```python
from build123d import *

# Parameters (mm, degrees)
BOSS_EXTRUDE1_DEPTH = 2
CHAMFER1_SIZE       = 0.3


with BuildPart() as part:
    # Sketch1 → Boss-Extrude1 (new body)
    with BuildSketch(Plane(origin=(0, 0, 0), x_dir=(0, 0, -1), z_dir=(1, 0, 0))):
        with BuildLine():
            Line((3.968626967, 0.5), (6.982120022, 0.5))
            ThreePointArc((6.982120022, 0.5), (-7, 0), (6.982120022, -0.5))
            Line((6.982120022, -0.5), (3.968626967, -0.5))
            ThreePointArc((3.968626967, -0.5), (-4, 0), (3.968626967, 0.5))
        make_face()
    extrude(amount=BOSS_EXTRUDE1_DEPTH)

    # Chamfer1
    chamfer1_edges = [part.edges().sort_by_distance(p)[0] for p in [
        (2, 0, 4),
        (2, 0, 7),
        (0, 0, 4),
        (0, 0, 7),
    ]]
    chamfer(chamfer1_edges, length=CHAMFER1_SIZE)


solid = part.part
```
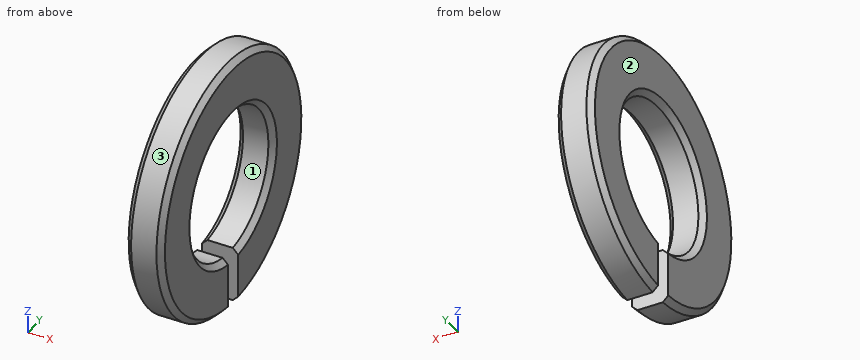
Source: CAD feature listing. Evaluate the final solid. Frame: model axes, mm. Face numbers are marked on the shaded views. Give positions to 0.01 mm unless a question says otherwise; leave off trailing zeros. Order: outer loops, then holes, each group sorted by start corner. A loop starts at its lowest first (then second) coordinate and runs counter-clockwise, first axis right, second up. Notation, with made-up numbers: (51.25, -12) -> (82.25, -12) arc R27 ccw to (82.25, 19) -> close; hole circle Ø4 at (7.25, 37.5). An arc over 180 degrees is marked (long way). Use a Markdown table: item, result.
Q1. Section A-A (z = 0). Return the cut outline in (x, y), and give its area (3 significant figures).
A:
| item | result |
|---|---|
| outline | (0, -6.7) -> (0.3, -7) -> (1.7, -7) -> (2, -6.7) -> (2, -4.3) -> (1.7, -4) -> (0.3, -4) -> (0, -4.3) -> close; (0, 4.3) -> (0.3, 4) -> (1.7, 4) -> (2, 4.3) -> (2, 6.7) -> (1.7, 7) -> (0.3, 7) -> (0, 6.7) -> close |
| area | 11.6 mm^2 |
Q2. Pull-direction query (Y, two-part tool) for the marked faces 1, 2 and 3; classes: +Y half, -Y half, draft (parallel to the pull), parting line (faces both ways), or undercut.
A:
| item | result |
|---|---|
| face 1 | undercut |
| face 2 | draft |
| face 3 | parting line |
Q3. Material intervals for line 1 (Y direction, x = 1, z = 0); line 2 (Y direction, x = 1.65, z = -1.25); line 3 (Z direction, x = 0.75, y = -6), sorted ascending. Write a range as [from, to].
A:
| item | result |
|---|---|
| line 1 | [-7, -4], [4, 7] |
| line 2 | [-6.89, -3.8], [3.8, 6.89] |
| line 3 | [-3.61, 3.61] |
Q4. Section B-B (y = 0). Return the cut outline in (x, z).
A:
| item | result |
|---|---|
| outline | (0, 4.3) -> (0.3, 4) -> (1.7, 4) -> (2, 4.3) -> (2, 6.7) -> (1.7, 7) -> (0.3, 7) -> (0, 6.7) -> close |
Q5. Section C-C (x = 1.2). Return the cut outline in (y, z).
A:
| item | result |
|---|---|
| outline | (-0.5, -6.98) -> (-0.5, -3.97) arc R4 cw (long way) to (0.5, -3.97) -> (0.5, -6.98) arc R7 ccw (long way) to start |
Q6. First-contact query: P1, Ø1, axis at x = 1, z = -6, coming from the +Y side. Flat tip, straight axial feed; report the tip coordinate or a pass-through.
A:
| item | result |
|---|---|
| P1 | y = 4.33 |
